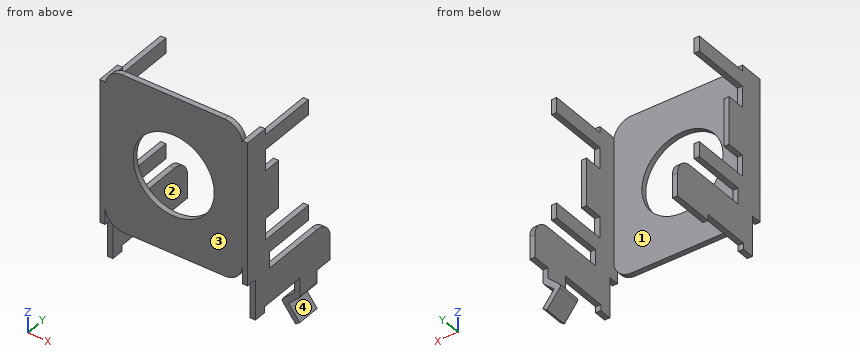
```python
from build123d import *

# Parameters (mm, degrees)
EXTRUDE003_DEPTH = 2
EXTRUDE001_DEPTH = 0.44
EXTRUDE_DEPTH    = 0.44
SKETCH027_R      = 3.4
EXTRUDE002_DEPTH = 0.44


with BuildPart() as extrude003:
    # Sketch028 → Extrude003 (new body)
    with BuildSketch(Plane.XZ):
        with BuildLine():
            Line((0, 0), (0, -1))
            ThreePointArc((0, -1), (0.027181, -1.129591), (0.104142, -1.237338))
            Line((0.104142, -1.237338), (0.941285, -2.007596))
            Line((0.941285, -2.007596), (0, -3.231801))
            Line((0, -3.231801), (0.348811, -3.5))
            Line((0.348811, -3.5), (1.43, -2.093841))
            ThreePointArc((1.43, -2.093841), (1.476737, -1.935298), (1.404702, -1.786533))
            Line((1.404702, -1.786533), (0.44, -0.885948))
            Line((0.44, -0.885948), (0.44, 0))
            Line((0.44, 0), (0, 0))
        make_face()
    extrude(amount=EXTRUDE003_DEPTH)


with BuildPart() as extrude003_1:
    # Extrude003 placement: moved
    add(extrude003.part.moved(Location((-6.2, 7.56, -3.4))))


with BuildPart() as part_mirroring:
    # Part__Mirroring: instance of Extrude003
    add(extrude003_1.part.mirror(Plane(origin=(0, 0, 0), x_dir=(0, -1, 0), z_dir=(1, 0, 0))))


with BuildPart() as extrude001:
    # Sketch026 → Extrude001 (new body)
    with BuildSketch(Plane.YZ):
        with BuildLine():
            Line((0, 12), (2.03, 12))
            Line((2.03, 12), (2.03, 11.5))
            Line((2.03, 11.5), (7, 11.5))
            Line((7, 11.5), (7, 10.24))
            Line((7, 10.24), (2.03, 10.24))
            Line((2.03, 10.24), (2.03, 8.44))
            Line((2.03, 8.44), (3.57, 8.44))
            Line((3.57, 8.44), (3.57, 4.44))
            Line((3.57, 4.44), (2.03, 4.44))
            Line((2.03, 4.44), (2.03, 2.64))
            Line((2.03, 2.64), (7, 2.64))
            Line((7, 2.64), (7, 1.38))
            Line((7, 1.38), (2.53, 1.38))
            Line((2.53, 1.38), (2.53, 0))
            Line((2.53, 0), (8, 0))
            ThreePointArc((9.5, -1.5), (9.06066, -0.43934), (8, 0))
            Line((9.5, -1.5), (9.5, -3.4))
            Line((9.5, -3.4), (6, -3.4))
            Line((6, -3.4), (6, -2.9))
            Line((6, -2.9), (1.93, -2.9))
            Line((1.93, -2.9), (1.93, -3.4))
            Line((1.93, -3.4), (0.9, -3.4))
            Line((0.9, -3.4), (0.9, 0))
            Line((0.9, 0), (0, 0))
            Line((0, 0), (0, 12))
        make_face()
    extrude(amount=EXTRUDE001_DEPTH)


with BuildPart() as extrude001_1:
    # Extrude001 placement: moved
    add(extrude001.part.moved(Location((5.76, -0.44, 0))))


with BuildPart() as fusion:
    # Sketch026 → Extrude (new body)
    with BuildSketch(Plane.YZ):
        with BuildLine():
            Line((0, 12), (2.03, 12))
            Line((2.03, 12), (2.03, 11.5))
            Line((2.03, 11.5), (7, 11.5))
            Line((7, 11.5), (7, 10.24))
            Line((7, 10.24), (2.03, 10.24))
            Line((2.03, 10.24), (2.03, 8.44))
            Line((2.03, 8.44), (3.57, 8.44))
            Line((3.57, 8.44), (3.57, 4.44))
            Line((3.57, 4.44), (2.03, 4.44))
            Line((2.03, 4.44), (2.03, 2.64))
            Line((2.03, 2.64), (7, 2.64))
            Line((7, 2.64), (7, 1.38))
            Line((7, 1.38), (2.53, 1.38))
            Line((2.53, 1.38), (2.53, 0))
            Line((2.53, 0), (8, 0))
            ThreePointArc((9.5, -1.5), (9.06066, -0.43934), (8, 0))
            Line((9.5, -1.5), (9.5, -3.4))
            Line((9.5, -3.4), (6, -3.4))
            Line((6, -3.4), (6, -2.9))
            Line((6, -2.9), (1.93, -2.9))
            Line((1.93, -2.9), (1.93, -3.4))
            Line((1.93, -3.4), (0.9, -3.4))
            Line((0.9, -3.4), (0.9, 0))
            Line((0.9, 0), (0, 0))
            Line((0, 0), (0, 12))
        make_face()
    extrude(amount=EXTRUDE_DEPTH)


with BuildPart() as fusion_1:
    # Extrude placement: moved
    add(fusion.part.moved(Location((-6.2, -0.44, 0))))

    # Fusion: union Extrude001
    add(extrude001_1.part)


with BuildPart() as metalcover:
    # Sketch027 → Extrude002 (new body)
    with BuildSketch(Plane.XZ):
        with BuildLine():
            Line((1.94, 13.2), (10.46, 13.2))
            ThreePointArc((11.96, 11.7), (11.52066, 12.76066), (10.46, 13.2))
            Line((11.96, 11.7), (11.96, 1.5))
            ThreePointArc((10.46, 0), (11.52066, 0.43934), (11.96, 1.5))
            Line((10.46, 0), (1.94, 0))
            ThreePointArc((0.44, 1.5), (0.87934, 0.43934), (1.94, 0))
            Line((0.44, 1.5), (0.44, 11.7))
            ThreePointArc((1.94, 13.2), (0.87934, 12.76066), (0.44, 11.7))
        make_face()
        with Locations((6.2, 6.6)):
            Circle(SKETCH027_R, mode=Mode.SUBTRACT)
    extrude(amount=EXTRUDE002_DEPTH)


with BuildPart() as metalcover_1:
    # Extrude002 placement: moved
    add(metalcover.part.moved(Location((-6.2, 0, 0))))

    # Fusion001: union Fusion
    add(fusion_1.part)

    # Fusion004: union Part__Mirroring
    add(part_mirroring.part)


solid = metalcover_1.part
```
Source: CAD feature listing. Evaluate the final solid. Frame: model axes, mm. Face numbers are marked on the shaded views. Give positions to 0.01 mm unless a question says otherwise; leave off trailing zeros. Order: outer loops, then holes, each group sorted by start corner. A loop starts at its lowest first (then second) coordinate and runs counter-clockwise, first axis right, second up.
(1) Material intervals for line 1 along Z through (x, y) = (0, -0.25); line 2 along X through (y, z) = (3.5, -1); line 3 along Y through (x, z) = (5, 9.5), sorted ascending.
(2) Section query C-C (z = 6.6). Return the cut outline in (x, y), plus the area to 3 significant figures.
(3) Contact query for flat-ended pins moving along their axis: P1, Ø0.5, axis at x = -6, z = 3.5, coming from the +Y side; P2, Ø0.5, axis at x = 6, y = 2.5, coming from the +Z side; P3, Ø3, axis at x = -1.5, z = 2, coming from the +Y side. Output: stop coordinate, or through.
(4) Section query A-A (y = 2.5). State how many separate pieces and enclosed holes the cut face has, plus the area to 3 significant figures.
(5) Pull-direction query (X, two-part tool) for the marked faces 1, 2, 3 and 4; classes: +X half, -X half, draft (parallel to the pull), parting line (faces both ways), or undercut.
(6) Section query B-B (x = 0). Return the cut outline in (y, z), plus the area to 3 significant figures.
(7) Section query D-D (y = 7.25). Return the cut outline in (x, z).
Outcome:
1. line 1: z = 0 to 3.2, 10 to 13.2
1. line 2: x = -6.2 to -5.76, 5.76 to 6.2
1. line 3: y = -0.44 to 0
2. outline: (-6.2, -0.44) - (-3.4, -0.44) - (-3.4, 0) - (-5.76, 0) - (-5.76, 3.13) - (-6.2, 3.13) - close; (3.4, -0.44) - (6.2, -0.44) - (6.2, 3.13) - (5.76, 3.13) - (5.76, 0) - (3.4, 0) - close
2. area: 5.22 mm2
3. P1: stops at y = 1.59
3. P2: stops at z = 11.5
3. P3: stops at y = 0
4. separate pieces: 8
4. enclosed holes: 0
4. area: 8.29 mm2
5. face 1: undercut
5. face 2: undercut
5. face 3: draft
5. face 4: +X half
6. outline: (-0.44, 0) - (0, 0) - (0, 3.2) - (-0.44, 3.2) - close; (-0.44, 10) - (0, 10) - (0, 13.2) - (-0.44, 13.2) - close
6. area: 2.82 mm2
7. outline: (-6.2, -3.4) - (-5.76, -3.4) - (-5.76, 0) - (-6.2, 0) - close; (4.77, -5.49) - (5.85, -6.9) - (6.2, -6.63) - (5.26, -5.41) - (6.1, -4.64) arc R0.32 ccw to (6.2, -4.4) - (6.2, 0) - (5.76, 0) - (5.76, -4.29) - (4.8, -5.19) arc R0.23 ccw to start
